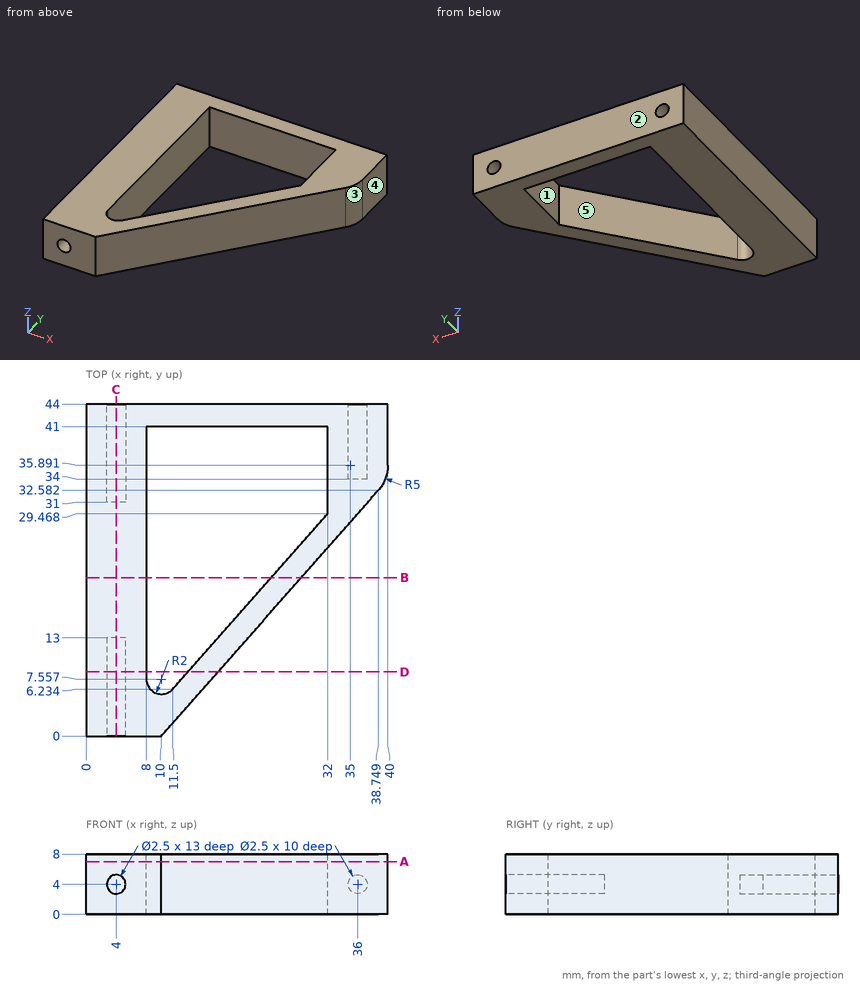
Geometry check sheet. Reference: drawing and pictorial views, mm from the part's lowest x, y, z. A direction names the side the tool comes from. Give positions to 0.01 mm unless a question says otherwise; leave off trailing zeros. Write each loop counter-clockwise with the first axis right and the second up, starting at its lowest first coordinate (ties: lowest second). Pieces come first, ordered by that corner, then holes.
Item 1: Gauge pin test, flat ends, axial feed: pin 1 (5 mm diameter, centred on x = 11.5, y = 37.5, fed in from +Z); pin 2 (4 mm diameter, centred on y = 21, z = 4, fed in from +X) (1 decimal); pin 3 (2 mm diameter, centred on x = 4, z = 4, fed in from +Y); pin 4 (1.5 mm diameter, centred on x = 11.5, z = 1.5, fed in from -Y). Record the tip position at first contact, or that the pin passes through.
Item 2: Cross-section at D-D (y = 8.5). Enter the section's corners in (x, z).
Item 3: Cross-section at A-A (z = 7). Enter the section's corners in (x, y).
Item 4: Access from +Z, -Z, +X, -X, +Y, -Y to the whole of each face (thin tool, end or side, straight path). Record for the marked faces 4 and 5.
Item 5: Scan lines: L1, parallel to Z at x = 4, y = 3.75; L2, parallel to X at y = 35, z = 4.75; L3, parallel to X at y = 37.5, z = 1.75. Record each from-to range of solid material in increasing order.
Item 6: Draft check along Y on the marked faces 1, 2 and 3. Enter one of: released by +Y, released by -Y, zero draft, split by the parting line, or undercut.
Item 7: Cross-section at B-B (y = 21). Enter the section's corners in (x, z).
Item 8: Cross-section at C-C (x = 4). Enter the section's corners in (y, z), and give its area (3 significant figures).
Report:
1. pin 1: passes through
1. pin 2: stops at x = 30.3
1. pin 3: stops at y = 31
1. pin 4: stops at y = 0.85
2. outline: (0, 0) - (8, 0) - (8, 8) - (0, 8) - close; (13.5, 0) - (17.5, 0) - (17.5, 8) - (13.5, 8) - close; hole circle Ø2.5 at (4, 4)
3. outline: (0, 0) - (10, 0) - (38.75, 32.58) arc R5 ccw to (40, 35.89) - (40, 44) - (0, 44) - close; hole (8, 7.56) arc R2 ccw to (11.5, 6.23) - (32, 29.47) - (32, 41) - (8, 41) - close
4. face 4: +Z, -Z, +X, +Y, -Y
4. face 5: +Z, -Z
5. L1: z = 0 to 2.75, 5.25 to 8
5. L2: x = 0 to 3, 5 to 8, 32 to 35, 37 to 39.92
5. L3: x = 0 to 8, 32 to 40
6. face 1: undercut
6. face 2: released by +Y
6. face 3: released by -Y
7. outline: (0, 0) - (8, 0) - (8, 8) - (0, 8) - close; (24.53, 0) - (28.53, 0) - (28.53, 8) - (24.53, 8) - close
8. outline: (0, 0) - (44, 0) - (44, 2.75) - (31, 2.75) - (31, 5.25) - (44, 5.25) - (44, 8) - (0, 8) - (0, 5.25) - (13, 5.25) - (13, 2.75) - (0, 2.75) - close
8. area: 287 mm2
